```python
from build123d import *

# Parameters (mm, degrees)
F1_DEPTH = 10
F3_DEPTH = 5


with BuildPart() as f1:
    # F0 (on Top) → F1 (new body)
    with BuildSketch(Plane.XY):
        Polygon((7.192049, 114.375856), (0, 114.440956), (0, -105.559044), (4.02688, -105.559044), (2.692049, -105.109864), (2.692049, -102.209864), (7.192049, -100.524144), (7.192049, -97.624144), (2.692049, -96.109864), (2.692049, -93.209864), (7.192049, -91.524144), (7.192049, -88.624144), (2.692049, -87.109864), (2.692049, -84.209864), (7.192049, -82.524144), (7.192049, -79.624144), (2.692049, -78.109864), (2.692049, -75.209864), (7.192049, -73.524144), (7.192049, -70.624144), (2.692049, -69.109864), (2.692049, -66.209864), (7.192049, -64.524144), (7.192049, -61.624144), (2.692049, -60.109864), (2.692049, -57.209864), (7.192049, -55.524144), (7.192049, -52.624144), (2.692049, -51.109864), (2.692049, -48.209864), (7.192049, -46.524144), (7.192049, -43.624144), (2.692049, -42.109864), (2.692049, -39.209864), (7.192049, -37.524144), (7.192049, -34.624144), (2.692049, -33.109864), (2.692049, -30.209864), (7.192049, -28.524144), (7.192049, -25.624144), (2.692049, -24.109864), (2.692049, -21.209864), (7.192049, -19.524144), (7.192049, -16.624144), (2.692049, -15.109864), (2.692049, -12.209864), (7.192049, -10.524144), (7.192049, -7.624144), (2.692049, -6.109864), (2.692049, -3.209864), (7.192049, -1.524144), (7.192049, 1.375856), (2.692049, 2.890136), (2.692049, 5.790136), (7.192049, 7.475856), (7.192049, 10.375856), (2.692049, 11.890136), (2.692049, 14.790136), (7.192049, 16.475856), (7.192049, 19.375856), (2.692049, 20.890136), (2.692049, 23.790136), (7.192049, 25.475856), (7.192049, 28.375856), (2.692049, 29.890136), (2.692049, 32.790136), (7.192049, 34.475856), (7.192049, 37.375856), (2.692049, 38.890136), (2.692049, 41.790136), (7.192049, 43.475856), (7.192049, 46.375856), (2.692049, 47.890136), (2.692049, 50.790136), (7.192049, 52.475856), (7.192049, 55.375856), (2.692049, 56.890136), (2.692049, 59.790136), (7.192049, 61.475856), (7.192049, 64.375856), (2.692049, 65.890136), (2.692049, 68.790136), (7.192049, 70.475856), (7.192049, 73.375856), (2.692049, 74.890136), (2.692049, 75.790136), (7.192049, 77.475856), (7.192049, 80.375856), (2.692049, 81.890136), (2.692049, 84.790136), (7.192049, 86.475856), (7.192049, 89.375856), (2.692049, 90.890136), (2.692049, 93.790136), (7.192049, 95.475856), (7.192049, 98.375856), (2.692049, 99.890136), (2.692049, 100.790136), (7.192049, 102.475856), (7.192049, 105.375856), (2.692049, 106.890136), (2.692049, 109.790136), (7.192049, 111.475856), align=None)
    extrude(amount=F1_DEPTH)

    # F2 (on face) → F3 (join)
    with BuildSketch(Plane(origin=(0, 0, 0), x_dir=(0, -1, 0), z_dir=(-1, 0, 0))):
        Polygon((-114.440956, 15), (-114.440956, 5), (-114.440956, -5), (105.559044, -5), (105.559044, 5), (105.559044, 15), align=None)
    extrude(amount=F3_DEPTH)


solid = f1.part
```
Read the model definition and answer for the solid it produces. Units are mm, in the model's axes. Give positions to 0.01 mm unless a question says otherwise; leave off trailing zeros. Loops run counter-clockwise (first coordinate to the right, second up) from the corner with the lowest first, then second, coordinate; pieces in that order, holes last.
Item 1: The part is cut by section A-A (z = 12). Write down the section's boundary in (x, y).
Item 2: Each of these flat-tipped pins is pushed along its axis until it touches: pin 1 Ø0.9 at (y, z) = (-14.5, 7) entering from +X; pin 2 Ø1.5 at (y, z) = (40.5, 13) entering from +X. Where does it stop, or does it pass through?
Item 3: The mould has two halves that part along Y. Classify faces 1 (the flat face through (-2, 114.441, 5)), 2 (the flat face through (-2, 3, 15)), 3 (the flat face through (4.91, -11.38, 4.93)): released by +Y, released by -Y, zero draft, split by the parting line, or undercut.
Item 4: Find the intervals of material crossed by line 1 along Z through (x, y) = (1, 78.5); line 2 along Y through (x, z) = (0.25, 8); line 3 along X through (y, z) = (75.5, 12.5), in increasing order.
Taken from the geometry:
1. outline: (-5, -105.56) - (0, -105.56) - (0, 114.44) - (-5, 114.44) - close
2. pin 1: stops at x = 2.69
2. pin 2: stops at x = 0
3. face 1: released by +Y
3. face 2: zero draft
3. face 3: undercut
4. line 1: z = 0 to 10
4. line 2: y = -105.56 to 114.44
4. line 3: x = -5 to 0
